Check sheet for the drawn part. Datum: minimum x, y, z corner. Units: mm. A direction names the side the tool comes from. Coordinates: 2 decimals unless noted, no trailing zeros. Loops run counter-clockwise (first coordinate to the right, second up) from the corner with the lowest first, then second, coordinate; pieces in that order, holes last.
Q1. Sectioned sample at B-B (y = 3). Enter the section's corners in (x, z), then the cut area to 3 significant figures.
Q2. Mould release check, pull along X, two halves, no side actions. Record for the marked faces 1, 2 and 3: +X half, -X half, draft (parallel to the pull), parting line (faces both ways), or undercut.
Q3. Sectioned sample at A-A (z = 12.75). Enter the section's corners in (x, y).
Q4. Access from +Z, -Z, +X, -X, +Y, -Y to the whole of each face (thin tool, end or side, straight path). Record for the marked faces 4, 5 and 6.
Q5. Material ranges on probe 1 along X at (y, z) = (23.5, 13.75); probe 2 along Z at (x, y) = (8, 22) (1 decimal); probe 3 along Y at (x, z) = (18, 7.5), recorded low to high.
Q6. Sectioned sample at C-C (y = 16). Enter the section's corners in (x, z) (1 decimal).
Q7. Sectioned sample at D-D (x = 8). Enter the section's corners in (y, z) (1 decimal).
Q8. Go/stop test with flat-tipped pins: P1, Ø1.5, axis at x = 14.5, z = 9, coming from the -Y side; P2, Ø3, axis at x = 4, y = 25.5, coming from the +Z side; P3, Ø3, axis at x = 11, y = 17.5, coming from the +Z side (1 decimal). Record where each tip stops, or that it passes through.
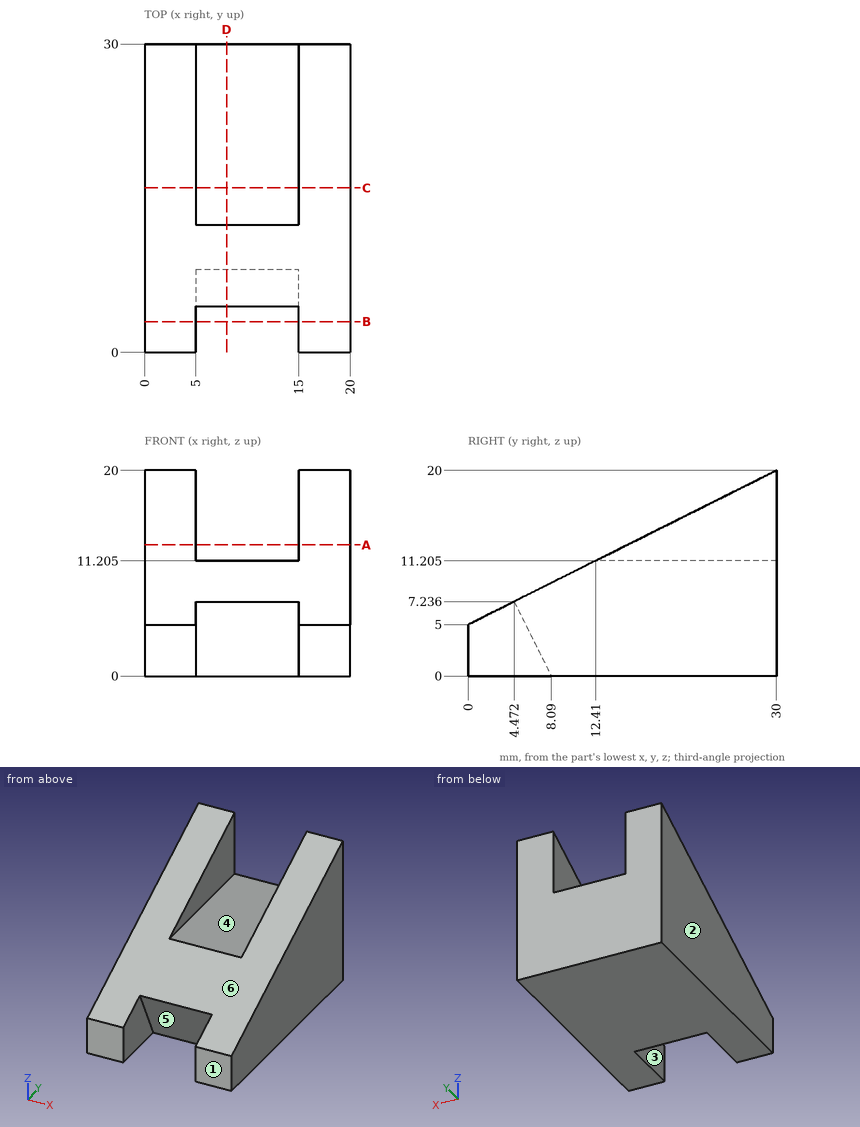
Geometry check:
1. outline: (0, 0) - (5, 0) - (5, 6.5) - (0, 6.5) - close; (15, 0) - (20, 0) - (20, 6.5) - (15, 6.5) - close
1. area: 65.0 mm2
2. face 1: draft
2. face 2: -X half
2. face 3: undercut
3. outline: (0, 15.5) - (5, 15.5) - (5, 30) - (0, 30) - close; (15, 15.5) - (20, 15.5) - (20, 30) - (15, 30) - close
4. face 4: +Z, +Y, -Y
4. face 5: -Z, -Y
4. face 6: +Z, +X, -X, -Y
5. probe 1: x = 0 to 5, 15 to 20
5. probe 2: z = 0 to 11.2
5. probe 3: y = 5 to 30
6. outline: (0, 0) - (20, 0) - (20, 13) - (15, 13) - (15, 11.2) - (5, 11.2) - (5, 13) - (0, 13) - close
7. outline: (4.5, 7.2) - (8.1, 0) - (30, 0) - (30, 11.2) - (12.4, 11.2) - close
8. P1: stops at y = 6.5
8. P2: stops at z = 18.5
8. P3: stops at z = 11.2
